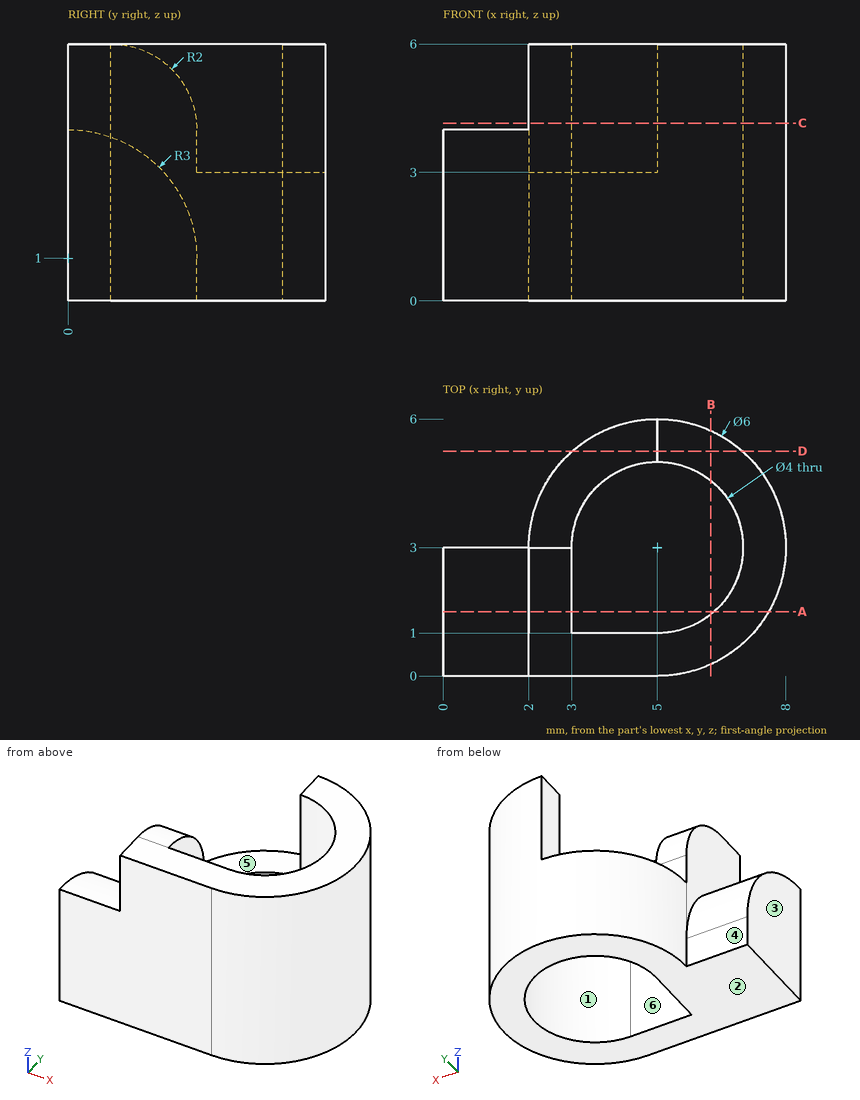
Design review of the part shown in the three views and the two pictorial views. Dimensions are in mm from the part's minimum x, y and z. A direction names the side the tool comes from. Coordinates: 2 decimals unless noted, no trailing zeros. Write each loop counter-clockwise with the first axis right and the second up, starting at its lowest first coordinate (ties: lowest second). Pieces come first, ordered by that corner, then holes.
1) We need section D-D on y = 5.25. State the section outline as (x, z) points, then the cut area to 3 significant figures.
2) We need section C-C on z = 4.15. State the section outline as (x, y) points, then the cut area to 3 significant figures.
3) To check wall thickness, follow probe 1 along X at (y, z) = (3, 1.6); probe 2 along Y at (x, z) = (1, 1.1); probe 3 along Y at (x, z) = (5.75, 5). State the ranges of each line that lie inside material, in increasing order.
4) We need section A-A on y = 1.5. State the section outline as (x, z) points.
5) We need section B-B on x = 6.25. State the section outline as (y, z) points, then the cut area to 3 significant figures.
6) Clearance check with flat-ended pins moving along their axes: pin 1 Ø0.6 at (y, z) = (1.5, 3.5) entering from +X; pin 2 Ø0.8 at (y, z) = (5.5, 5) entering from -X; pin 3 Ø0.8 at (x, z) = (2.5, 3.5) entering from +Y. State where each tip first meets the part, or that it passes through.
7) The part is to be moulded in two halves that separate along X. For the marked faces 1, 2 and 3, say which applies: pulls with the +X half, pulls with the -X half, needs draft (parallel to the pull), parting line crosses it, or undercut.
8) Machinability: for the marked faces 4, 5 and 6, which of the approach directions +Z, -Z, +X, -X, +Y, -Y give a long, thin tool a straight path to every point of the face, cutting with its end or side? Answer none if there is none.
Answer list:
1. outline: (3.02, 0) - (6.98, 0) - (6.98, 6) - (5, 6) - (5, 3) - (3.02, 3) - close
1. area: 17.9 mm2
2. outline: (2, 0) - (5, 0) arc R3 ccw to (5, 6) - (5, 5) arc R2 cw to (5, 1) - (3, 1) - (3, 2.99) - (2, 2.99) - close
2. area: 12.8 mm2
3. probe 1: x = 2 to 3, 7 to 8
3. probe 2: y = 0 to 3
3. probe 3: y = 0.1 to 1.15, 4.85 to 5.9
4. outline: (0, 0) - (3, 0) - (3, 5.94) - (2, 5.94) - (2, 3.6) - (0, 3.6) - close; (6.32, 0) - (7.6, 0) - (7.6, 6) - (6.32, 6) - close
5. outline: (0.27, 0) - (1.44, 0) - (1.44, 6) - (0.27, 6) - close; (4.56, 0) - (5.73, 0) - (5.73, 6) - (4.56, 6) - close
5. area: 14.0 mm2
6. pin 1: stops at x = 7.75
6. pin 2: stops at x = 5
6. pin 3: stops at y = 3
7. face 1: undercut
7. face 2: needs draft
7. face 3: pulls with the -X half
8. face 4: +Z, -Z, -X, +Y
8. face 5: +Z, -X, +Y
8. face 6: +Z, -Z
